Read the model definition and answer for the solid it produces. Units are mm, in the model's axes. A direction names the side the tool comes from. Coordinates: 2 decimals unless noted, no trailing zeros. Order: outer loops, then holes, each group sorted by start corner. A loop starts at its lowest first (then second) coordinate and runs counter-clockwise, first axis right, second up. Notation, with made-up numbers: (59.25, 59) - (85.25, 59) arc R12 ccw to (85.25, 77) - close; hole circle Ø6 at (-4, 10). An arc over 180 degrees is marked (long way). Write item = value, one per line.
from build123d import *

# Parameters (mm, degrees)
CROQUIS1_W              = 41
CROQUIS1_H              = 55
SALIENTE_EXTRUIR1_DEPTH = 6
CROQUIS2_W              = 35
CROQUIS2_H              = 55
CORTAR_EXTRUIR1_DEPTH   = 3
REDONDEO1_R             = 2
CROQUIS3_W              = 10
CROQUIS3_H              = 10
CORTAR_EXTRUIR2_DEPTH   = 3


with BuildPart() as part:
    # Croquis1 → Saliente-Extruir1 (new body)
    with BuildSketch(Plane.XY):
        with Locations((-72.407619756, 7.664233577)):
            Rectangle(CROQUIS1_W, CROQUIS1_H)
    extrude(amount=SALIENTE_EXTRUIR1_DEPTH)

    # Croquis2 → Cortar-Extruir1 (cut)
    with BuildSketch(Plane.XY.offset(6)):
        with Locations((-72.407619756, 7.664233577)):
            Rectangle(CROQUIS2_W, CROQUIS2_H)
    extrude(amount=-CORTAR_EXTRUIR1_DEPTH, mode=Mode.SUBTRACT)

    # Redondeo1
    # the kernel refuses this fillet: 2 mm, written as the material it takes off along each edge
    with BuildSketch(Plane(origin=(-54.907619756, 40.164233577, 6), x_dir=(1, 0, 0), z_dir=(0, -1, 0)), Plane(origin=(-51.907619756, 40.164233577, 6), x_dir=(0, 0, -1), z_dir=(0, -1, 0)), Plane(origin=(-51.907619756, 40.164233577, 0), x_dir=(-1, 0, 0), z_dir=(0, -1, 0)), Plane(origin=(-92.907619756, -24.835766423, 0), x_dir=(1, 0, 0), z_dir=(0, 1, 0))) as redondeo1_piece_1:
        with BuildLine():
            CenterArc((REDONDEO1_R, -REDONDEO1_R), REDONDEO1_R, 90, 90)
            Line((0, -REDONDEO1_R), (0, 0))
            Line((0, 0), (REDONDEO1_R, 0))
        make_face()
    extrude(amount=65, mode=Mode.SUBTRACT)
    with BuildSketch(Plane(origin=(-92.907619756, -24.835766423, 6), x_dir=(1, 0, 0), z_dir=(0, 1, 0)), Plane(origin=(-89.907619756, -24.835766423, 6), x_dir=(0, 0, -1), z_dir=(0, 1, 0))) as redondeo1_piece_2:
        with BuildLine():
            CenterArc((REDONDEO1_R, REDONDEO1_R), REDONDEO1_R, 180, 90)
            Line((0, REDONDEO1_R), (0, 0))
            Line((0, 0), (REDONDEO1_R, 0))
        make_face()
    extrude(amount=65, mode=Mode.SUBTRACT)

    # Croquis3 → Cortar-Extruir2 (cut)
    with BuildSketch(Plane(origin=(0, 0, 0), x_dir=(-1, 0, 0), z_dir=(0, 0, -1))):
        with Locations((81.907619756, -10.335766423)):
            Rectangle(CROQUIS3_W, CROQUIS3_H)
        with Locations((62.907619756, -10.335766423)):
            Rectangle(CROQUIS3_W, CROQUIS3_H)
        with Locations((62.907619756, 7.664233577)):
            Rectangle(CROQUIS3_W, CROQUIS3_H)
        with Locations((62.907619756, 25.664233577)):
            Rectangle(CROQUIS3_W, CROQUIS3_H)
        with Locations((81.907619756, 7.664233577)):
            Rectangle(CROQUIS3_W, CROQUIS3_H)
        with Locations((81.907619756, 25.664233577)):
            Rectangle(CROQUIS3_W, CROQUIS3_H)
    extrude(amount=-CORTAR_EXTRUIR2_DEPTH, mode=Mode.SUBTRACT)


solid = part.part
1) The part is cut by section D-D (z = 4.65). Determine the outline of the cut face in (x, y), and give its area (3 significant figures).
Returned:
outline = (-92.8, -19.84) - (-90.02, -19.84) - (-90.02, 35.16) - (-92.8, 35.16) - close; (-54.8, -19.84) - (-52.02, -19.84) - (-52.02, 35.16) - (-54.8, 35.16) - close
area = 306 mm^2
2) The part is cut by section A-A (y = -12). Determine the outline of the cut face in (x, z), and give its area (3 significant figures).
Returned:
outline = (-92.91, 2) arc R2 ccw to (-90.91, 0) - (-86.91, 0) - (-86.91, 3) - (-89.91, 3) - (-89.91, 4) arc R2 ccw to (-91.41, 5.94) arc R2 ccw to (-92.91, 4) - close; (-76.91, 0) - (-67.91, 0) - (-67.91, 3) - (-76.91, 3) - close; (-57.91, 0) - (-53.91, 0) arc R2 ccw to (-51.91, 2) - (-51.91, 4) arc R2 ccw to (-53.41, 5.94) arc R2 ccw to (-54.91, 4) - (-54.91, 3) - (-57.91, 3) - close
area = 75.9 mm^2
3) Determine the mould class of faces 4 (the face through (-54.477, 8.049, 5.239)), 5 (the face through (-86.908, 26, 1)), 6 (the face through (-82, -5.336, 1)), 7 (the face through (-73, -19.836, 2)) for opening direction Y: pulls with the +Y half, pulls with the -Y half, needs draft (parallel to the pull), parting line crosses it, or undercut.
Returned:
face_4 = needs draft
face_5 = undercut
face_6 = undercut
face_7 = pulls with the -Y half
4) For faces 1 (the face through (-51.908, 7, 3)), 2 (the face through (-90.34, 7.28, 5.24)), 3 (the face through (-76.908, -10, 1)), determine the directions among +Z, -Z, +X, -X, +Y, -Y from which every point of the face is accessible in a straight line to the end or side of a thin tool.
Returned:
face_1 = +Z, -Z, +X, +Y, -Y
face_2 = +Z, +Y, -Y
face_3 = +Z, -Z
5) The part is cut by section C-C (z = 0.65). Determine the outline of the cut face in (x, y).
Returned:
outline = (-92.38, -19.84) - (-52.43, -19.84) - (-52.43, 35.16) - (-92.38, 35.16) - close; hole (-86.91, -15.34) - (-76.91, -15.34) - (-76.91, -5.34) - (-86.91, -5.34) - close; hole (-86.91, 2.66) - (-76.91, 2.66) - (-76.91, 12.66) - (-86.91, 12.66) - close; hole (-86.91, 20.66) - (-76.91, 20.66) - (-76.91, 30.66) - (-86.91, 30.66) - close; hole (-67.91, -15.34) - (-57.91, -15.34) - (-57.91, -5.34) - (-67.91, -5.34) - close; hole (-67.91, 2.66) - (-57.91, 2.66) - (-57.91, 12.66) - (-67.91, 12.66) - close; hole (-67.91, 20.66) - (-57.91, 20.66) - (-57.91, 30.66) - (-67.91, 30.66) - close
6) The part is cut by section B-B (x = -79). Determine the outline of the cut face in (y, z), and give its area (3 significant figures).
Returned:
outline = (-19.84, 0) - (-15.34, 0) - (-15.34, 3) - (-19.84, 3) - close; (-5.34, 0) - (2.66, 0) - (2.66, 3) - (-5.34, 3) - close; (12.66, 0) - (20.66, 0) - (20.66, 3) - (12.66, 3) - close; (30.66, 0) - (35.16, 0) - (35.16, 3) - (30.66, 3) - close
area = 75.0 mm^2
7) Flat-ended cylindrical pins translate along their axes: pin 1 Ø0.9 at (y, z) = (6, 1) entering from -X; pin 2 Ø1.5 at (y, z) = (9, 1) entering from -X; pin 3 Ø10.5 at (x, y) = (-74.5, -4.5) entering from +Z. Find the tip coordinate at first contact, or state that the pin passes through.
Returned:
pin_1 = -92.83
pin_2 = -92.89
pin_3 = 3
8) Straight lines are drawn through the part: line 1 along Y through (x, z) = (-64, 0.3); line 2 along X through (y, z) = (-12, 2.5); line 3 along X through (y, z) = (29, 3.7). For each, find the intervals that lie inside material, in ascending order. Write a range as from..to.
Returned:
line_1 = -19.84..-15.34, -5.34..2.66, 12.66..20.66, 30.66..35.16
line_2 = -92.91..-86.91, -76.91..-67.91, -57.91..-51.91
line_3 = -92.91..-89.91, -54.91..-51.91
